Read the model definition and answer for the solid it produces. Units are mm, in the model's axes. Coordinates: 2 decimals unless noted, no trailing zeros. Write each loop counter-clockwise with the first axis right and the second up, starting at its lowest first coordinate (ties: lowest second). Pieces come first, ordered by that corner, then holes.
Autodesk Inventor part; units mm, degrees
ref_plane "YZ Plane" through (0, 0, 0) normal (1, 0, 0) x (0, 1, 0)
ref_plane "XZ Plane" through (0, 0, 0) normal (0, 1, 0) x (-1, 0, 0)
ref_plane "Work Plane1" through (0, 0, 0.5) normal (0, 0, 1) x (1, 0, 0)
sketch "Sketch1" plane through (0, 0, 0.5) normal (0, 0, 1) x (1, 0, 0)
  arc A0 (4.1391, 2.5087) -> (3.9017, 2.864) centre (0, 0) ccw construction
  arc A1 (1.2602, 4.4787) -> (2.2758, 4.058) centre (1.7603, 4.2498) ccw construction
  circle A2 centre (0, 0) radius 4.05 construction
  circle A3 centre (284.3339, -363.0367) radius 11 construction
  circle A4 centre (483.573, -598.8165) radius 11 construction
  circle A5 centre (41.6311, -972.2671) radius 11 construction
  circle A6 centre (-157.608, -736.4873) radius 11 construction
  line L0 (110.2354, -491.8247) -> (106.3399, -495.1165) construction
  line L1 (108.2876, -493.4706) -> (162.0638, -557.1094) construction
  line L2 (110.2239, -495.762) -> (-164.7078, -728.0854)
  line L3 (-166.0099, -743.5871) -> (33.2292, -979.3669)
  line L4 (48.7309, -980.669) -> (490.6728, -607.2184)
  line L5 (492.0682, -591.8285) -> (3.1278, 2.5728)
  arc A7 (3.1278, 2.5728) -> (-3.0968, -2.6101) centre (0, 0) ccw
  arc A8 (-164.7078, -728.0854) -> (-166.0099, -743.5871) centre (-157.608, -736.4873) ccw
  arc A9 (33.2292, -979.3669) -> (48.7309, -980.669) centre (41.6311, -972.2671) ccw
  arc A10 (490.6728, -607.2184) -> (492.0682, -591.8285) centre (483.573, -598.8165) ccw
  circle A11 centre (284.3339, -363.0367) radius 12.5 construction
  line L6 (292.4019, -372.5844) -> (125.3917, -513.7116)
  line L7 (-3.0968, -2.6101) -> (293.8919, -354.981)
  arc A12 (292.4019, -372.5844) -> (293.8919, -354.981) centre (284.3339, -363.0367) ccw
  line L8 (124.4236, -512.5659) -> (291.4337, -371.4387)
  arc A13 (291.4337, -371.4387) -> (292.7449, -355.9477) centre (284.3339, -363.0367) ccw
  line L9 (292.7449, -355.9477) -> (-4.2437, -3.5768)
  arc A14 (4.2862, 3.5257) -> (-4.2437, -3.5768) centre (0, 0) ccw
  line L10 (4.2862, 3.5257) -> (493.2266, -590.8756)
  arc A15 (491.641, -608.3641) -> (493.2266, -590.8756) centre (483.573, -598.8165) ccw
  line L11 (491.641, -608.3641) -> (49.6991, -981.8147)
  arc A16 (32.0835, -980.335) -> (49.6991, -981.8147) centre (41.6311, -972.2671) ccw
  line L12 (32.0835, -980.335) -> (-167.1556, -744.5553)
  arc A17 (-165.6759, -726.9396) -> (-167.1556, -744.5553) centre (-157.608, -736.4873) ccw
  line L13 (-165.6759, -726.9396) -> (109.2558, -494.6163)
  line L14 (125.3917, -513.7116) -> (124.4236, -512.5659)
  line L15 (109.2558, -494.6163) -> (110.2239, -495.762)
  point P0 (0, 0)
extrude "Extrusion1" add sketch "Sketch1" along normal blind 6
equation "\"d2\" = d1"
properties part number "Belt1"
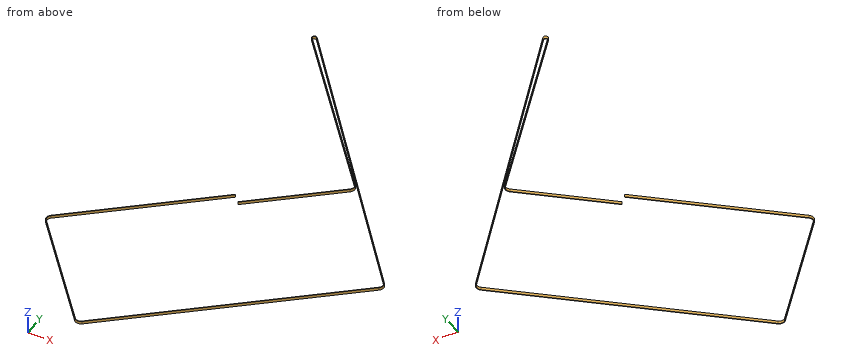
Item 1: Find the intervals of material crossed by probe 1 along Y at (x, z) = (283.5, 6.15); probe 2 along Y at (x, z) = (231, 1.75); probe 3 along Y at (x, z) = (367, 1.55), in increasing order.
Item 2: The part is cut by section A-A (y = -550.5). Give the vertices of the cut face in (x, z).
Item 3: The part is cut by section C-C (x = 445). Give the vertices of the cut face in (y, z).
Item 4: The part is cut by section B-B (z = 5.1). Give the vertices of the cut face in (x, y) (1 decimal), and give its area (3 significant figures).
Item 5: The part is cut by section D-D (x = 176.5). Give the vertices of the cut face in (y, z), and give its area (3 significant figures).
Item 6: Given pin 1 (3 mm diameter, centred on y = -692, z = 3, fed in from -X); pin 2 (3 mm diameter, centred on x = 383.5, z = 2.5, fed in from +Y), each flat-ended and moving along its own axis, determine where each tip first touches the part or whether it passes through.
Answer:
1. probe 1: y = -784.25 to -782.28, -380.11 to -378.14, -344.98 to -342.65, -338.27 to -335.91
1. probe 2: y = -828.61 to -826.65, -424.47 to -422.51, -282.69 to -280.36, -274.45 to -272.09
1. probe 3: y = -713.69 to -711.72, -439.78 to -437.42
2. outline: (43.12, 0.5) - (45.45, 0.5) - (45.45, 6.5) - (43.12, 6.5) - close; (458.07, 0.5) - (460.01, 0.5) - (460.01, 6.5) - (458.07, 6.5) - close
3. outline: (-647.78, 0.5) - (-645.81, 0.5) - (-645.81, 6.5) - (-647.78, 6.5) - close; (-534.61, 0.5) - (-532.25, 0.5) - (-532.25, 6.5) - (-534.61, 6.5) - close
4. outline: (-167.2, -744.6) - (32.1, -980.3) arc R12.5 ccw to (49.7, -981.8) - (491.6, -608.4) arc R12.5 ccw to (493.2, -590.9) - (4.3, 3.5) arc R5.5 ccw (long way) to (-4.2, -3.6) - (292.7, -355.9) arc R11 cw to (291.4, -371.4) - (124.4, -512.6) - (125.4, -513.7) - (292.4, -372.6) arc R12.5 ccw to (293.9, -355) - (-3.1, -2.6) arc R4.1 cw (long way) to (3.1, 2.6) - (492.1, -591.8) arc R11 cw to (490.7, -607.2) - (48.7, -980.7) arc R11 cw to (33.2, -979.4) - (-166, -743.6) arc R11 cw to (-164.7, -728.1) - (110.2, -495.8) - (109.3, -494.6) - (-165.7, -726.9) arc R12.5 ccw to start
4. area: 4,180 mm2
5. outline: (-874.67, 0.5) - (-872.7, 0.5) - (-872.7, 6.5) - (-874.67, 6.5) - close; (-470.52, 0.5) - (-468.56, 0.5) - (-468.56, 6.5) - (-470.52, 6.5) - close; (-218.03, 0.5) - (-215.7, 0.5) - (-215.7, 6.5) - (-218.03, 6.5) - close; (-208.19, 0.5) - (-205.83, 0.5) - (-205.83, 6.5) - (-208.19, 6.5) - close
5. area: 51.7 mm2
6. pin 1: stops at x = -126.1
6. pin 2: stops at y = -455.66
